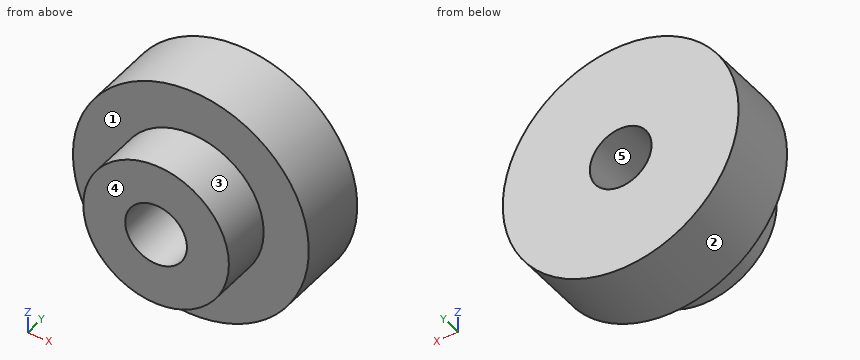
Autodesk Inventor part; units mm, degrees
ref_plane "YZ Plane" through (0, 0, 0) normal (1, 0, 0) x (0, 1, 0)
ref_plane "XZ Plane" through (0, 0, 0) normal (0, 1, 0) x (-1, 0, 0)
ref_plane "XY Plane" through (0, 0, 0) normal (0, 0, 1) x (1, 0, 0)
sketch "Sketch1" plane through (0, 0, 0) normal (0, 1, 0) x (-1, 0, 0)
  circle A0 centre (0, 0) radius 7.45
  dimension "d0" = 14.9
extrude "Extrusion1" add sketch "Sketch1" along normal blind 7.9
sketch "Sketch2" plane through (0, 0, 0) normal (0, 1, 0) x (-1, 0, 0)
  circle A0 centre (0, 0) radius 4.6
  circle A1 centre (0, 0) radius 7.45
  dimension "d3" = 9.2
extrude "Extrusion2" cut sketch "Sketch2" along normal blind 3.3
sketch "Sketch3" plane through (0, 7.9, 0) normal (0, 1, 0) x (1, 0, 0)
  point P0 (0, 0)
  point P1 (0, 0)
hole "Hole1" at (0, 7.9, 0) direction (0, -1, 0) diameter 3.9 end through all
properties part number "HeadBarClampTurnwheel" material "UHMW, White"
Read the model definition and answer for the solid it produces. Units are mm, in the model's axes. Face numbers are marked on the shaded views. A direction names the side the tool comes from. Round coordinates to 2 decimals unless told otherwise and drop trailing zeros. Loops run counter-clockwise (first coordinate to the right, second up) from the corner with the lowest first, then second, coordinate; pieces in that order, holes last. Notation, with made-up numbers: (87.5, 24.5) - (143.5, 24.5) arc R25 cw to (143.5, 59.5) - close; hole circle Ø4 at (63, 43.5). An arc over 180 degrees is marked (long way). One line per question, with ' | ' between items. Start each with the question number.
Q1. Section C-C on y = 1.75 is taken. Give the vertices of the cut face in (x, z).
Q2. Find the intervals of material crossed by L1, parallel to Z at x = 0, y = 4.75; L2, parallel to Z at x = 0, y = 3; L3, parallel to Y at x = 3.5, z = -4.5, in increasing order.
Q3. Flat-ended cylindrical pins translate along their axes: pin 1 (3 mm diameter, centred on x = -2, z = -0.5, fed in from -Y); pin 2 (2 mm diameter, centred on y = 2, z = -1.5, fed in from -X); pin 3 (1.5 mm diameter, centred on x = 6, z = -2, fed in from -Y); pin 4 (1.5 mm diameter, centred on y = 2.5, z = 2.5, fed in from -X). Find the tip coordinate at first contact, or state that the pin passes through.
Q4. For the marked faces 1 and 2, determine the directions among +Z, -Z, +X, -X, +Y, -Y from which every point of the face is accessible in a straight line to the end or side of a thin tool.
Q5. Section D-D on x = 2.75 is taken. Give the vertices of the cut face in (y, z), plus the area to 3 significant figures.
Q6. Section B-B on x = 0 is taken. Give the vertices of the cut face in (y, z), plus the area to 3 significant figures.
Q7. For a pull along Z with two mould halves and no side action, classify the marked faces 3, 4 and 5 as +Z half, -Z half, draft (parallel to the pull), parting line (faces both ways), or undercut.
Q8. Section A-A on z = 0 is taken. Give the vertices of the cut face in (x, y).
Established:
1) outline: circle Ø9.2 at (0, 0); hole circle Ø3.9 at (0, 0)
2) L1: -7.45 to -1.95, 1.95 to 7.45 | L2: -4.6 to -1.95, 1.95 to 4.6 | L3: 3.3 to 7.9
3) pin 1: y = 0 | pin 2: x = -4.57 | pin 3: y = 3.3 | pin 4: x = -4.25
4) face 1: -Y | face 2: +Y, -Y
5) outline: (0, -3.69) - (3.3, -3.69) - (3.3, -6.92) - (7.9, -6.92) - (7.9, 6.92) - (3.3, 6.92) - (3.3, 3.69) - (0, 3.69) - close | area: 88.0 mm²
6) outline: (0, -4.6) - (3.3, -4.6) - (3.3, -7.45) - (7.9, -7.45) - (7.9, -1.95) - (0, -1.95) - close; (0, 1.95) - (7.9, 1.95) - (7.9, 7.45) - (3.3, 7.45) - (3.3, 4.6) - (0, 4.6) - close | area: 68.1 mm²
7) face 3: parting line | face 4: draft | face 5: undercut
8) outline: (-7.45, 3.3) - (-4.6, 3.3) - (-4.6, 0) - (-1.95, 0) - (-1.95, 7.9) - (-7.45, 7.9) - close; (1.95, 0) - (4.6, 0) - (4.6, 3.3) - (7.45, 3.3) - (7.45, 7.9) - (1.95, 7.9) - close
